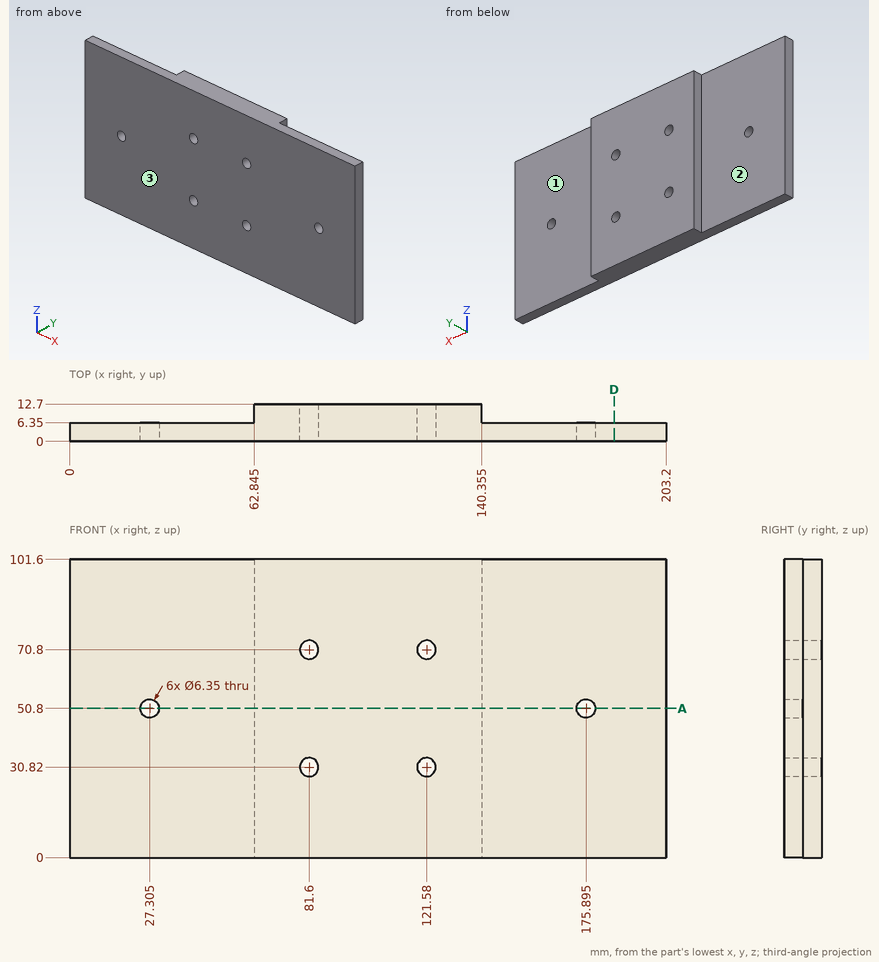
Input: dimensioned drawing with shaded views. Units: mm. Origin: part minimum x, y, z. A direction names the side the tool comes from. Coordinates: 2 decimals unless noted, no trailing zeros. Loops run counter-clockwise (first coordinate to the right, second up) from the corner with the lowest first, then second, coordinate; pieces in that order, holes last.
Q1. Section A-A, the plane z = 50.8. Give the number of separate pieces and of enclosed holes in the cut face, and give its area (3 significant figures).
Results are:
separate pieces: 3
enclosed holes: 0
area: 1,700 mm2
Q2. Line query: line 1 along Z through (x, y) = (80.5, 6); line 2 along X through (y, z) = (0.5, 73.5); line 3 along X through (y, z) = (2.75, 69) (1 decimal). Output: solid intervals per line, ascending.
Results are:
line 1: z = 0 to 27.84, 33.8 to 67.82, 73.78 to 101.6
line 2: x = 0 to 79.93, 83.27 to 119.91, 123.25 to 203.2
line 3: x = 0 to 79, 84.2 to 119, 124.2 to 203.2
Q3. Contact query for flat-ended pins moving along their axis: pin 1 (3 mm diameter, centred on x = 22.5, z = 23, fed in from +Y); pin 2 (1.5 mm diameter, centred on y = 8.5, z = 63, fed in from -X) (3 decimals); pin 3 (5.5 mm diameter, centred on x = 81.6, z = 70.8, fed in from +Y); pin 4 (1.5 mm diameter, centred on y = 10.5, z = 72.5, fed in from +X) (3 decimals). Output: stop coordinate, or through.
Results are:
pin 1: stops at y = 6.35
pin 2: stops at x = 62.845
pin 3: passes through
pin 4: stops at x = 140.355
Q4. Section D-D, the plane x = 185.5. Return the cut outline in (y, z), and give its area (3 significant figures).
Results are:
outline: (0, 0) - (6.35, 0) - (6.35, 101.6) - (0, 101.6) - close
area: 645 mm2
Q5. Set-up query: the marked faces 1, 2 and 3. Return all of +Z, -Z, +X, -X, +Y, -Y with unobstructed straight access to the full face (end or side cutting, diameter ignored); none if empty.
Results are:
face 1: +Z, -Z, +X, +Y
face 2: +Z, -Z, -X, +Y
face 3: +Z, -Z, +X, -X, -Y
